from build123d import *

# Parameters (mm, degrees)
SKETCH_3_W          = 40
SKETCH_3_H          = 20
EXTRUDE_3_DEPTH     = 100
SKETCH_4_W          = 40
SKETCH_4_H          = 20
SKETCH_4_W_2        = 31.6
SKETCH_4_H_2        = 11.6
CUT_EXTRUDE_1_DEPTH = 20


with BuildPart() as part:
    # 草图3 → 凸台-拉伸3 (new body)
    with BuildSketch(Plane.XY):
        Rectangle(SKETCH_3_W, SKETCH_3_H)
    extrude(amount=EXTRUDE_3_DEPTH)

    # 草图4 → 切除-拉伸1 (cut)
    with BuildSketch(Plane.XY.offset(100)):
        Rectangle(SKETCH_4_W, SKETCH_4_H)
        Rectangle(SKETCH_4_W_2, SKETCH_4_H_2, mode=Mode.SUBTRACT)
    extrude(amount=-CUT_EXTRUDE_1_DEPTH, mode=Mode.SUBTRACT)


solid = part.part
Verification items for the finished model (mm, model axes). A direction names the side the tool comes from. Give positions to 0.01 mm unless a question says otherwise; leave off trailing zeros. Write each loop counter-clockwise with the first axis right and the second up, starting at its lowest first coordinate (ties: lowest second). Pieces come first, ordered by that corner, then holes. Notation, with made-up numbers: (0, 64) - (47, 64) arc R27 ccw to (47, 88) - close; hole circle Ø8 at (84.25, -10). An arc over 180 degrees is marked (long way). Answer as CSV lines item,"result". Start each with the question number.
1. Thickness scan on line 1 (Z direction, x = 2, y = 8.75). Record the ranges inside material, lowest first.
2. Depth check by flat-ended pin: pin 1 (6 mm diameter, centred on x = -7.5, z = 91.5, fed in from -Y); pin 2 (3.5 mm diameter, centred on y = 1.5, z = 85.5, fed in from +X); pin 3 (16 mm diameter, centred on x = 5, z = 88.5, fed in from +Y). Enter the tip coordinate at first touch or a pass-through.
3. Sectioned sample at B-B (x = 8.5). Record the boundary of the cut face in (y, z), then the cut area to 3 significant figures.
4. Sectioned sample at A-A (y = 4.75). Record the boundary of the cut face in (x, z).
5. Set-up check for faces 1 (the face through (0, 5.8, 90)), 2 (the face through (-15.8, 0, 90)), 3 (the face through (0, -5.8, 90)), 4 (the face through (15.8, 0, 90)): record each of +Z, -Z, +X, -X, +Y, -Y from which the full face is reachable in a straight line by a thin tool's end or side.
Derived:
1,line 1,"0 to 80"
2,pin 1,"y = -5.8"
2,pin 2,"x = 15.8"
2,pin 3,"y = 5.8"
3,outline,"(-10, 0) - (10, 0) - (10, 80) - (5.8, 80) - (5.8, 100) - (-5.8, 100) - (-5.8, 80) - (-10, 80) - close"
3,area,"1,830 mm²"
4,outline,"(-20, 0) - (20, 0) - (20, 80) - (15.8, 80) - (15.8, 100) - (-15.8, 100) - (-15.8, 80) - (-20, 80) - close"
5,face 1,"+Z, +X, -X, +Y"
5,face 2,"+Z, -X, +Y, -Y"
5,face 3,"+Z, +X, -X, -Y"
5,face 4,"+Z, +X, +Y, -Y"
